from build123d import *

# Parameters (mm, degrees)
F1_DEPTH = 15.875
F2_W     = 19.05
F2_H     = 12.7
F3_DEPTH = 25.4
F4_R     = 7.874
F5_DEPTH = 25.4


with BuildPart() as f1:
    # F0 (on Front) → F1 (new body, symmetric)
    with BuildSketch(Plane.XZ):
        Polygon((0, 12.7), (0, 0), (47.752, 0), (54.102, 22.352), (88.9, 22.352), (88.9, 35.052), (44.45, 35.052), (38.1, 12.7), align=None)
    extrude(amount=F1_DEPTH, both=True)

    # F2 (on face) → F3 (cut)
    with BuildSketch(Plane.XY.offset(35.052)):
        with Locations((79.375, 0)):
            Rectangle(F2_W, F2_H)
    extrude(amount=-F3_DEPTH, mode=Mode.SUBTRACT)

    # F4 (on face) → F5 (cut)
    with BuildSketch(Plane.XY.offset(12.7)):
        with Locations((19.05, 0)):
            Circle(F4_R)
    extrude(amount=-F5_DEPTH, mode=Mode.SUBTRACT)


solid = f1.part
Can you work these out from the model? Positions are in its coordinate system, mm. A direction names the side the tool comes from. Coordinates: 2 decimals unless noted, no trailing zeros. Loops run counter-clockwise (first coordinate to the right, second up) from the corner with the lowest first, then second, coordinate; pieces in that order, holes last. Notation, with made-up numbers: M 73,54 L 121,54 A15 cw 121,76 Z; hole C -29,4 d5. An arc over 180 degrees is marked long. Answer as CSV lines item,"result". Start each with the question number.
1. Suppose I cut it at A-A, the plane x = 19.05. List the corners of the cut face in (y, z) for me (3 decimals), plus the area to 3 significant figures.
2. Suppose I cut it at C-C, the plane z = 3.5. List the corners of the cut face in (x, y) for me (3 decimals).
3. If I drill on probe 1 along Y at (x, z) = (78, 31.5) (3 decimals); probe 2 along Y at (x, z) = (19, 4) (3 decimals); probe 3 along Z at (x, y) = (7.5, 1), over which ranges is the centre line in solid material (lowest first)? Write a range as [from, to].
4. Suppose I cut it at D-D, the plane y = -10.5. List the corners of the cut face in (x, z) for me, plus the area to 3 significant figures.
5. For faces 1 (the face through (67, 0, 22.352)), 2 (the face through (88.9, 11, 29)), 3 (the face through (24, -7, 12.7)), 4 (the face through (79, -6.35, 29)), which set-ups out of +Z, -Z, +X, -X, +Y, -Y let a thin tool reach every point of the face, with its end or its side?
6. For pin 1 Ø9.5 at (x, y) = (25.5, 5.5) entering from +Z; pin 2 Ø4 at (y, z) = (-1.5, 30.5) entering from +X; pin 3 Ø3 at (y, z) = (11.5, 16.5) entering from +X, each with a flat end and sliding along its axis, tell me the tip position at first contact or that it passes through.
7. Suppose I cut it at B-B, the plane y = 0. List the corners of the cut face in (x, z) for me, plus the area to 3 significant figures.
8. Thinking about a two-plate mould opening in Y: for faces 5 (the face through (44, 15.875, 18)), 6 (the face through (50.883, -0.222, 11.02)), 7 (the face through (11.184, 0.346, 6.439)), 8 (the face through (69.85, 0, 29)), which applies, +Y half, -Y half, draft (parallel to the pull), parting line (faces both ways), or undercut?
Output:
1,outline,"M -15.875,0 L -7.874,0 L -7.874,12.7 L -15.875,12.7 Z; M 7.874,0 L 15.875,0 L 15.875,12.7 L 7.874,12.7 Z"
1,area,"203 mm^2"
2,outline,"M 0,-15.875 L 48.746,-15.875 L 48.746,15.875 L 0,15.875 Z; hole C 19.05,0 d15.748"
3,probe 1,"y = [-15.875, -6.35], [6.35, 15.875]"
3,probe 2,"y = [-15.875, -7.874], [7.874, 15.875]"
3,probe 3,"z = [0, 12.7]"
4,outline,"M 0,0 L 47.75,0 L 54.1,22.35 L 88.9,22.35 L 88.9,35.05 L 44.45,35.05 L 38.1,12.7 L 0,12.7 Z"
4,area,"1,340 mm^2"
5,face 1,"-Z, +X, +Y, -Y"
5,face 2,"+Z, -Z, +X, +Y, -Y"
5,face 3,"+Z, -X, +Y, -Y"
5,face 4,"+Z, -Z, +X"
6,pin 1,"stops at z = 12.7"
6,pin 2,"stops at x = 69.85"
6,pin 3,"stops at x = 52.87"
7,outline,"M 0,0 L 11.18,0 L 11.18,12.7 L 0,12.7 Z; M 26.92,0 L 47.75,0 L 54.1,22.35 L 69.85,22.35 L 69.85,35.05 L 44.45,35.05 L 38.1,12.7 L 26.92,12.7 Z"
7,area,"903 mm^2"
8,face 5,"+Y half"
8,face 6,"draft"
8,face 7,"undercut"
8,face 8,"undercut"
